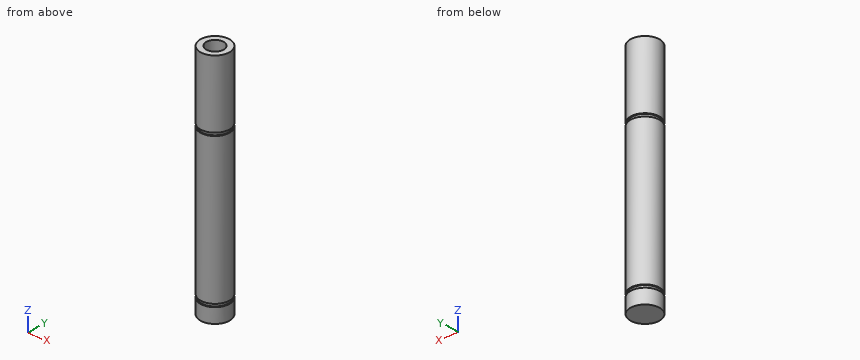
Autodesk Inventor part; units mm, degrees
ref_plane "YZ Plane" through (0, 0, 0) normal (1, 0, 0) x (0, 1, 0)
ref_plane "XZ Plane" through (0, 0, 0) normal (0, 1, 0) x (-1, 0, 0)
ref_plane "XY Plane" through (0, 0, 0) normal (0, 0, 1) x (1, 0, 0)
sketch "Sketch2" plane through (0, 0, 0) normal (0, 0, 1) x (1, 0, 0)
  circle A0 centre (0, 0) radius 5
  dimension "d0" = 10
extrude "Extrusion1" add sketch "Sketch2" against normal blind 80
sketch "Sketch3" plane through (0, 0, 0) normal (0, 1, 0) x (-1, 0, 0)
  line L0 (-5, -80) -> (5, -80)
  line L1 (5, 0) -> (-5, 0)
  point P0 (0, 0)
sketch "Sketch4" plane through (0, 0, 0) normal (0, 1, 0) x (-1, 0, 0)
  line L0 (-5, 0) -> (-5, -80)
  line L1 (-5, -75) -> (-4.6, -75)
  line L2 (-4.6, -75) -> (-4.6, -74)
  line L3 (-4.6, -74) -> (-5, -74)
  line L4 (-5, -74) -> (-5, -75)
  line L5 (-5, -80) -> (5, -80)
  line L6 (0, -96) -> (0, 16)
  point P0 (0, 0)
  point P1 (-5, -74)
  dimension "d3" = 5
  dimension "d4" = 1
  dimension "d5" = 0.4
revolve "Revolution1" cut sketch "Sketch4" angle 360 about axis through (0, 0, 0) along (0, 0, 1)
sketch "Sketch5" plane through (0, 0, 0) normal (0, 1, 0) x (-1, 0, 0)
  line L0 (-5, 0) -> (-5, -74)
  line L1 (-5, -24) -> (-4.6, -24)
  line L2 (-4.6, -24) -> (-4.6, -23)
  line L3 (-4.6, -23) -> (-5, -23)
  line L4 (-5, -23) -> (-5, -24)
  line L5 (5, -74) -> (-5, -74)
  line L6 (0, -96) -> (0, 16)
  point P0 (0, 0)
  point P1 (-5, -23)
  dimension "d7" = 50
  dimension "d8" = 1
  dimension "d9" = 0.4
revolve "Revolution2" cut sketch "Sketch5" angle 360 about axis through (0, 0, 0) along (0, 0, 1)
sketch "Sketch7" plane through (0, 0, 0) normal (0, 0, 1) x (1, 0, 0)
  circle A0 centre (0, 0) radius 3
  dimension "d11" = 6
extrude "Extrusion2" cut sketch "Sketch7" against normal blind 10
equation "\"BendRadius\" = Thickness"
equation "\"BendReliefWidth\" = Thickness"
equation "\"BendReliefDepth\" = 0.5 * Thickness"
equation "\"CornerReliefSize\" = 4 * Thickness"
equation "\"MinimumRemnant\" = 2 * Thickness"
equation "\"TransitionRadius\" = BendRadius"
equation "\"JacobiRadiusSize\" = BendRadius"
equation "\"GapSize\" = Thickness"
properties part number "Shaft_potentiometer"
CAD build for the part. Positions are in the model's coordinates, mm. Give positions to 0.01 mm unless a question says otherwise; leave off trailing zeros. Write each loop counter-clockwise with the first axis right and the second up, starting at its lowest first coordinate (ties: lowest second). Pieces come first, ordered by that corner, then holes. Notation, with made-up numbers: (72, -26) - (100, -26) arc R30 cw to (100, 10) - close; hole circle Ø6 at (47, 0.5). An arc over 180 degrees is marked (long way). Put each result on its own line as item: value.
(1) Drop flat-ended pins along their axis: pin 1 Ø1.5 at (x, y) = (0.5, 1.5) entering from +Z; pin 2 Ø3 at (x, z) = (-3, -42.5) entering from +Y; pin 3 Ø1.5 at (x, z) = (-4, -55.5) entering from +Y. Give the stop position or say it passes through.
Working result:
pin 1: z = -10
pin 2: y = 4.77
pin 3: y = 3.8
(2) Saw through at A-A (x = 0). List the corners of the cut face in (y, z), then the cut area to 3 significant figures.
Working result:
outline: (-5, -80) - (5, -80) - (5, -75) - (4.6, -75) - (4.6, -74) - (5, -74) - (5, -24) - (4.6, -24) - (4.6, -23) - (5, -23) - (5, 0) - (3, 0) - (3, -10) - (-3, -10) - (-3, 0) - (-5, 0) - (-5, -23) - (-4.6, -23) - (-4.6, -24) - (-5, -24) - (-5, -74) - (-4.6, -74) - (-4.6, -75) - (-5, -75) - close
area: 738 mm^2
(3) Saw through at C-C (z = -6). List the corners of the cut face in (x, y).
Working result:
outline: circle Ø10 at (0, 0); hole circle Ø6 at (0, 0)
(4) Wall check: L1, parallel to Z at x = 3.5, y = -3.25; L2, parallel to Y at x = 0, z = -8; L3, parallel to X at y = 0.25, z = -14. Give the ranges that are in metal, low to high.
Working result:
L1: -80 to -75, -74 to -24, -23 to 0
L2: -5 to -3, 3 to 5
L3: -4.99 to 4.99
(5) Saw through at D-D (z = -38). List the corners of the cut face in (x, y), then the cut area to 3 significant figures.
Working result:
outline: circle Ø10 at (0, 0)
area: 78.5 mm^2
